Part model, mm, in its own coordinate system. Face numbers are marked on the shaded views. A direction names the side the tool comes from. Round coordinates to 2 decimals unless told otherwise and drop trailing zeros. Write each loop counter-clockwise with the first axis right and the second up, starting at its lowest first coordinate (ties: lowest second). Pieces come first, ordered by that corner, then holes.
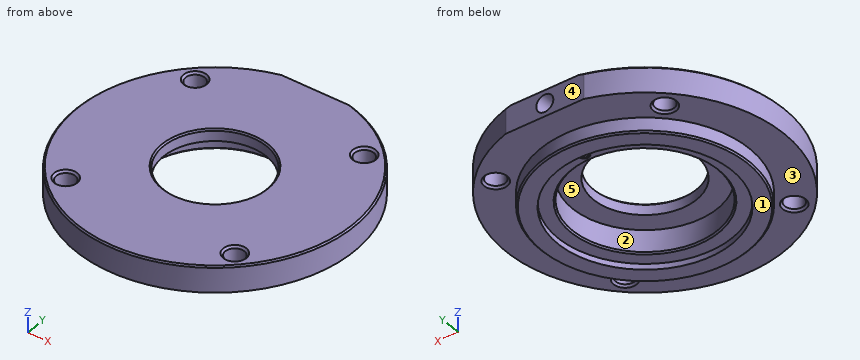
```python
from build123d import *

# Parameters (mm, degrees)
CIRPATTERN1_COUNT               = 4
SKETCH4_W                       = 93.853238467
SKETCH4_H                       = 20.664933241
CUT_EXTRUDE1_DEPTH              = 69.476273263
F_3_0MM_DOWEL_HOLE1_D           = 3
F_3_0MM_DOWEL_HOLE1_DEPTH       = 9.098709071
F_3_0MM_DOWEL_HOLE1_CSINK_D     = 3.5
F_3_0MM_DOWEL_HOLE1_CSINK_ANGLE = 90
F_3_0MM_DOWEL_HOLE1_TIP         = 0.901290929


with BuildPart() as part:
    # Sketch1 → Revolve1 (revolve)
    with BuildSketch(Plane(origin=(0, 0, 0), x_dir=(0, 0, -1), z_dir=(1, 0, 0)), mode=Mode.PRIVATE) as revolve1_sk:
        Polygon((0, -18.25), (0, -47.5), (0.5, -48), (9, -48), (9, -36), (13.5, -36), (14, -35.5), (14, -30), (12, -30), (12, -25.5), (11.5, -25), (4, -25), (4, -17.75), (0.5, -17.75), align=None)
    revolve(revolve1_sk.sketch.rotate(Axis((0, 0, 0), (0, 0, -1)), 270), axis=Axis((0, 0, 0), (0, 0, -1)))

    # Sketch3 → Ø6.0mm Dowel Hole1 (revolve, cut)
    with BuildSketch(Plane(origin=(-29.69848481, 29.69848481, -9), x_dir=(0, 1, 0), z_dir=(1, 0, 0))):
        Polygon((0, 0), (0, 9), (4, 9), (3.3, 8.3), (3.3, 0.7), (4, 0), align=None)
    f_6_0mm_dowel_hole1 = revolve(axis=Axis((-29.69848481, 29.69848481, -15.35), (0, 0, 1)), mode=Mode.SUBTRACT)

    # CirPattern1: Ø6.0mm Dowel Hole1 ×4 about axis
    cirpattern1_axis = Axis((0, 0, 0), (0, 0, 1))
    for i in range(1, CIRPATTERN1_COUNT):
        add(f_6_0mm_dowel_hole1.rotate(cirpattern1_axis, i * 360 / CIRPATTERN1_COUNT), mode=Mode.SUBTRACT)

    # Sketch4 → Cut-Extrude1 (cut, through all)
    with BuildSketch(Plane(origin=(0, 0, -9), x_dir=(-1, 0, 0), z_dir=(0, 0, -1))):
        with Locations((-0.198842092, 56.33246662)):
            Rectangle(SKETCH4_W, SKETCH4_H)
    extrude(amount=-CUT_EXTRUDE1_DEPTH, mode=Mode.SUBTRACT)

    # Ø3.0mm Dowel Hole1
    with Locations(Plane(origin=(0, 0, -12), x_dir=(-1, 0, 0), z_dir=(0, 0, -1))):
        with Locations((0, 28)):
            CounterSinkHole(F_3_0MM_DOWEL_HOLE1_D / 2, F_3_0MM_DOWEL_HOLE1_CSINK_D / 2, depth=F_3_0MM_DOWEL_HOLE1_DEPTH, counter_sink_angle=F_3_0MM_DOWEL_HOLE1_CSINK_ANGLE)
            with Locations((0, 0, -(F_3_0MM_DOWEL_HOLE1_DEPTH + F_3_0MM_DOWEL_HOLE1_TIP / 2))):  # 118° drill point
                Cone(0, F_3_0MM_DOWEL_HOLE1_D / 2, F_3_0MM_DOWEL_HOLE1_TIP, mode=Mode.SUBTRACT)

    # Sketch9 → Hole1 (revolve, cut)
    with BuildSketch(Plane(origin=(0, 46, -4.5), x_dir=(0, 0, 1), z_dir=(1, 0, 0))):
        Polygon((0, 0), (0, 18), (1.5, 17.098709071), (1.5, 7.901290929), (3, 7), (3, 0), align=None)
    revolve(axis=Axis((0, 52.130023899, -4.5), (0, -1, 0)), mode=Mode.SUBTRACT)


solid = part.part
```
Q1. Which spindle directions (+Z, -Z, +X, -X, +Y, -Y) get a long thin tool onto all of the face, cutting with end or side? Do the marked faces 1 and 2. Say none if no direction does.
Values follow:
face 1: -Z, +X, -X, +Y, -Y
face 2: -Z
Q2. Cut at A-A on y = 0. Write the cut outline in (x, z).
Values follow:
outline: (-48, -9) - (-36, -9) - (-36, -13.5) - (-35.5, -14) - (-30, -14) - (-30, -12) - (-25.5, -12) - (-25, -11.5) - (-25, -4) - (-17.75, -4) - (-17.75, -0.5) - (-18.25, 0) - (-47.5, 0) - (-48, -0.5) - close; (17.75, -4) - (25, -4) - (25, -11.5) - (25.5, -12) - (30, -12) - (30, -14) - (35.5, -14) - (36, -13.5) - (36, -9) - (48, -9) - (48, -0.5) - (47.5, 0) - (18.25, 0) - (17.75, -0.5) - close
Q3. Wall check: L1, parallel to X at y = 0.5, z = -11.5 (3 decimals); L2, parallel to Y at x = -30.5, z = -8; L3, parallel to Y at x = -31, z = -3. Give the ranges that are in metal, low to high.
Values follow:
L1: x = -35.997 to -24.995, 24.995 to 35.997
L2: y = -37.06 to -32.9, -26.5 to 26.5, 32.9 to 37.06
L3: y = -36.65 to -32.73, -26.67 to 26.67, 32.73 to 36.65
Q4. Drop flat-ended pins along their axis: pin 1 (4 mm diameter, centred on x = -29.7, y = 29.7, fed in from -Z); pin 2 (8 mm diameter, centred on y = 34, z = -10.5, fed in from +X); pin 3 (1.5 mm diameter, centred on y = -5, z = -4, fed in from +X); pin 4 (1 mm diameter, centred on x = 5.5, z = -3, fed in from -Y). Give the stop position or say it passes through.
Values follow:
pin 1: passes through
pin 2: stops at x = 37.23
pin 3: stops at x = 47.81
pin 4: stops at y = -47.74
Q5. Mould opens along Y. For the marked faces 3, 4 and 5 say: +Y half, -Y half, draft (parallel to the pull), parting line (faces both ways), or undercut.
Values follow:
face 3: draft
face 4: +Y half
face 5: undercut
